The drawing under review shows one solid part. Ordinate dimensions are in mm from its lowest x, y, z. A direction names the side the tool comes from. Give positions to 0.01 mm unless a question says otherwise; leave off trailing zeros. Loops run counter-clockwise (first coordinate to the right, second up) from the corner with the lowest first, then second, coordinate; pieces in that order, holes last. Notation, with made-up numbers: (42.5, 31) -> (78.5, 31) arc R22 cw to (78.5, 61) -> close; hole circle Ø3 at (-30, 16). An arc over 180 degrees is marked (long way). Answer in a Markdown table with one row per item. Add a question column.
(1) For line 1 (Z direction, x = 33, y = 41.2); line 2 (Y direction, x = 16, z = 6); line 3 (X direction, y = 13.5, z = 7.5), list the stretches that pass through material, from the lowest coordinate up.
(2) For pin 1 (2 mm diameter, centred on x = 33, z = 5, fed in from -Y), flat-tipped, find the tip position at first contact; note if it passes through.
(3) Consider section B-B on y = 22.5. Write out the cut boundary in (x, z).
(4) Consider section C-C on x = 24.5. Write out the cut boundary in (y, z).
(5) For the marked faces 1 and 2, list the 3-axis set-ups (+Z, -Z, +X, -X, +Y, -Y) from which the entire face can be reached by the end or side of a thin tool; tool diameter is ignored.
(6) Draft analysis for pull direction Y (two halves, no side actions). For the marked faces 3, 4, 5 and 6, state which applies: +Y half, -Y half, draft (parallel to the pull), parting line (faces both ways), or undercut.
(7) Consider section A-A on z = 5. Write out the cut boundary in (x, y).
(8) Consider section D-D on z = 8.5. Write out the cut boundary in (x, y).
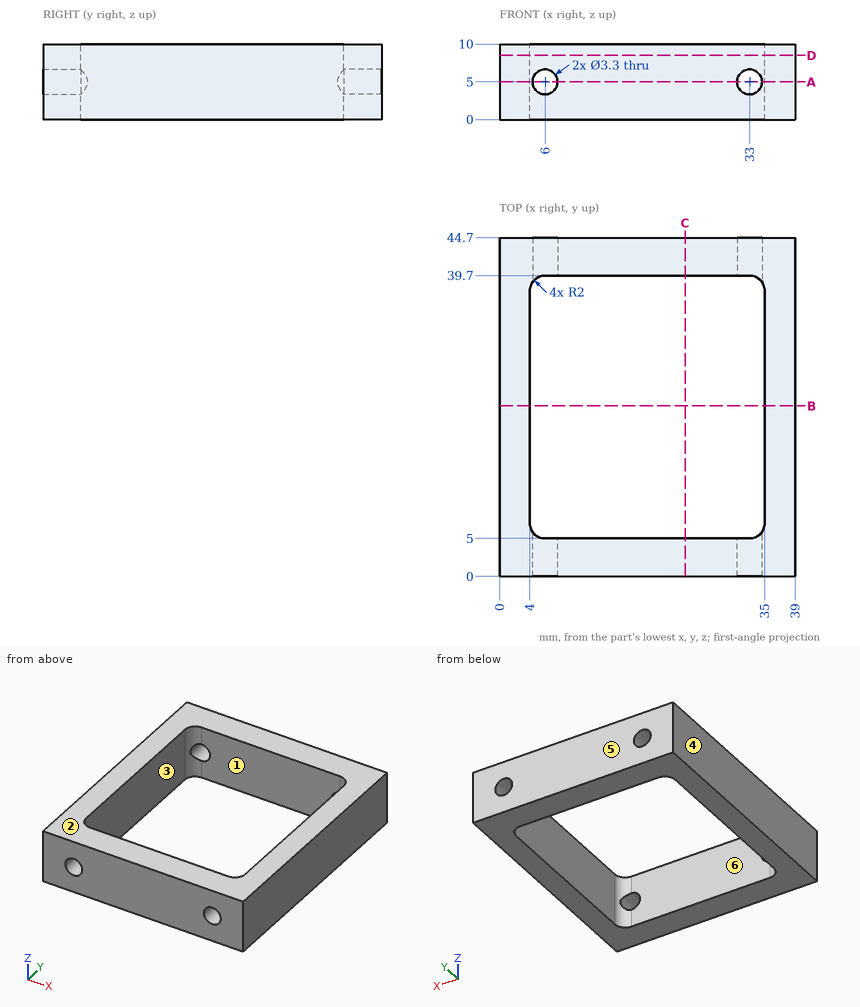
Values follow:
| question | item | result |
|---|---|---|
| 1 | line 1 | 0 to 3.35, 6.65 to 10 |
| 1 | line 2 | 0 to 5, 39.7 to 44.7 |
| 1 | line 3 | 0 to 4, 35 to 39 |
| 2 | pin 1 | through |
| 3 | outline | (0, 0) -> (4, 0) -> (4, 10) -> (0, 10) -> close; (35, 0) -> (39, 0) -> (39, 10) -> (35, 10) -> close |
| 4 | outline | (0, 0) -> (5, 0) -> (5, 10) -> (0, 10) -> close; (39.7, 0) -> (44.7, 0) -> (44.7, 10) -> (39.7, 10) -> close |
| 5 | face 1 | +Z, -Z |
| 5 | face 2 | +Z, +X, -X, +Y, -Y |
| 6 | face 3 | undercut |
| 6 | face 4 | draft |
| 6 | face 5 | +Y half |
| 6 | face 6 | undercut |
| 7 | outline | (0, 0) -> (4.35, 0) -> (4.35, 5.87) arc R2 cw to (4, 7) -> (4, 37.7) arc R2 cw to (4.35, 38.83) -> (4.35, 44.7) -> (0, 44.7) -> close; (7.65, 0) -> (31.35, 0) -> (31.35, 5) -> (7.65, 5) -> close; (7.65, 39.7) -> (31.35, 39.7) -> (31.35, 44.7) -> (7.65, 44.7) -> close; (34.65, 0) -> (39, 0) -> (39, 44.7) -> (34.65, 44.7) -> (34.65, 38.83) arc R2 cw to (35, 37.7) -> (35, 7) arc R2 cw to (34.65, 5.87) -> close |
| 8 | outline | (0, 0) -> (39, 0) -> (39, 44.7) -> (0, 44.7) -> close; hole (4, 7) arc R2 ccw to (6, 5) -> (33, 5) arc R2 ccw to (35, 7) -> (35, 37.7) arc R2 ccw to (33, 39.7) -> (6, 39.7) arc R2 ccw to (4, 37.7) -> close |
